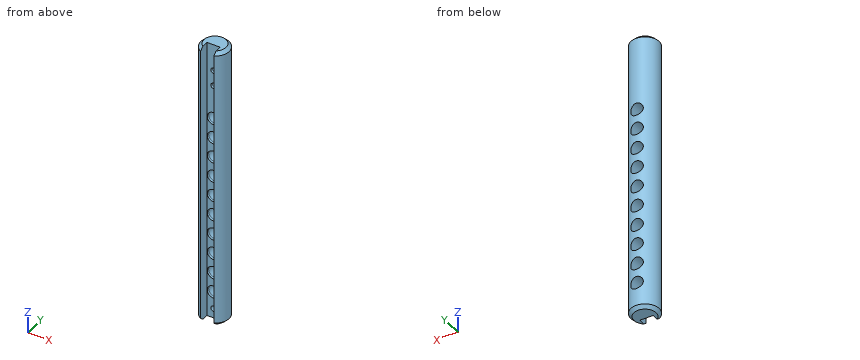
from build123d import *

# Parameters (mm, degrees)
PAD_DEPTH            = 180
CHAMFER_SIZE         = 2
SKETCH001_R          = 4
POCKET_DEPTH         = 7.960899
POCKET_DEPTH_BACK    = 9.001
SKETCH016_R          = 1.75
POCKET008_DEPTH      = 4
BODY_PLACEMENT_ANGLE = 180


with BuildPart() as part:
    # Sketch → Pad (new body)
    with BuildSketch(Plane.XY):
        with BuildLine():
            ThreePointArc((-4.2, 7.959899), (0, -9), (4.2, 7.959899))
            Line((4.2, 1.459899), (4.2, 7.959899))
            Line((-4.2, 1.459899), (4.2, 1.459899))
            Line((-4.2, 7.959899), (-4.2, 1.459899))
        make_face()
    extrude(amount=PAD_DEPTH)

    # Chamfer
    chamfer_edges = [part.edges().sort_by_distance(p)[0] for p in [
        (0, -9, 180),
        (0, -9, 0),
    ]]
    chamfer(chamfer_edges, length=CHAMFER_SIZE)

    # Sketch001 → Pocket (cut, two sides)
    with BuildSketch(Plane.XZ) as pocket_sk:
        with Locations((0, 17)):
            Circle(SKETCH001_R)
        with Locations((0, 29.7)):
            Circle(SKETCH001_R)
        with Locations((0, 42.4)):
            Circle(SKETCH001_R)
        with Locations((0, 55.1)):
            Circle(SKETCH001_R)
        with Locations((0, 67.8)):
            Circle(SKETCH001_R)
        with Locations((0, 80.5)):
            Circle(SKETCH001_R)
        with Locations((0, 93.2)):
            Circle(SKETCH001_R)
        with Locations((0, 105.9)):
            Circle(SKETCH001_R)
        with Locations((0, 118.6)):
            Circle(SKETCH001_R)
        with Locations((0, 131.3)):
            Circle(SKETCH001_R)
    extrude(amount=-POCKET_DEPTH, mode=Mode.SUBTRACT)
    extrude(pocket_sk.sketch, amount=POCKET_DEPTH_BACK, mode=Mode.SUBTRACT)

    # Sketch016 → Pocket008 (cut, symmetric)
    with BuildSketch(Plane.XZ):
        with Locations((0, 162.900868)):
            Circle(SKETCH016_R)
        with Locations((0, 152.900868)):
            Circle(SKETCH016_R)
        with Locations((0, 6)):
            Circle(SKETCH016_R)
    extrude(amount=POCKET008_DEPTH, both=True, mode=Mode.SUBTRACT)


with BuildPart() as part_1:
    # Body placement: moved
    add(part.part.moved(Location((0, -15, -37.5))).rotate(Axis((0, -15, -37.5), (0, 0, 1)), BODY_PLACEMENT_ANGLE))


solid = part_1.part
Geometry check sheet. Reference: the model listing, model coordinates, mm. Round coordinates to 2 decimals unless told otherwise and drop trailing zeros. Order: outer loops, then holes, each group sorted by start corner. A loop starts at its lowest first (then second) coordinate and runs counter-clockwise, first axis right, second up. Notation, with made-up numbers: M 39.25,-16.75 L 71.25,-16.75 A16 ccw 71.25,-1.75 Z; hole C 45,-11.5 d2. An arc over 180 degrees is marked long. Answer in a Markdown table with one row per item. Add a question column.
Item 1: Sectioned sample at D-D, the plane z = 10.5. Enter the section's corners in (x, y).
Item 2: Sectioned sample at B-B, the plane x = 0. State how many separate pieces and enclosed holes the cut face has, plus the area to 3 significant figures.
Item 3: Depth check by flat-ended pin: pin 1 Ø9 at (x, z) = (0, 4.9) entering from +Y; pin 2 Ø2 at (x, z) = (0, 115.4) entering from -Y; pin 3 Ø7 at (y, z) = (-19, 35.5) entering from +X; pin 4 Ø3 at (x, z) = (-5.5, 114) entering from +Y. Enter the tip coordinate at first touch or a pass-through.
Item 4: Sectioned sample at A-A, the plane z = 43. Enter the section's corners in (x, y), plus the area to 3 significant figures.
Item 5: Sectioned sample at C-C, the plane z = -31.5. Enter the section's corners in (x, y), plus the area to 3 significant figures.
Item 6: Material ranges on L1, parallel to X at y = -15, z = 20; L2, parallel to X at y = -9.75, z = 68.4; L3, parallel to Y at x = -0.25, z = 49.5, recorded low to high. Write a range as [from, to].
Filled in:
| question | item | result |
|---|---|---|
| 1 | outline | M -4.2,-22.96 L -4.2,-16.46 L 4.2,-16.46 L 4.2,-22.96 A9 ccw long Z |
| 2 | separate pieces | 11 |
| 2 | enclosed holes | 0 |
| 2 | area | 985 mm² |
| 3 | pin 1 | stops at y = -6 |
| 3 | pin 2 | stops at y = -11 |
| 3 | pin 3 | stops at x = 8.99 |
| 3 | pin 4 | stops at y = -6.94 |
| 4 | outline | M -4.2,-22.96 L -4.2,-16.46 L -4,-16.46 L -4,-6.94 A9 ccw Z; M 4,-16.46 L 4.2,-16.46 L 4.2,-22.96 A9 ccw 4,-6.94 Z |
| 4 | area | 113 mm² |
| 5 | outline | M -4.2,-22.96 L -4.2,-16.46 L -1.75,-16.46 L -1.75,-11 L 1.75,-11 L 1.75,-16.46 L 4.2,-16.46 L 4.2,-22.96 A9 ccw long Z |
| 5 | area | 175 mm² |
| 6 | L1 | x = [-9, -3.2], [3.2, 9] |
| 6 | L2 | x = [-7.31, -4], [4, 7.31] |
| 6 | L3 | y = [-16.46, -6] |
